Here's how the part is built. I have some questions about the finished solid (model axes, mm). Coordinates: 2 decimals unless noted, no trailing zeros. Write each loop counter-clockwise with the first axis right and the second up, starting at its lowest first coordinate (ties: lowest second). Pieces come first, ordered by that corner, then holes. Notation, with made-up numbers: (2.25, 32.25) - (23.25, 32.25) arc R12 cw to (23.25, 37.25) - close; hole circle Ø10 at (25, 4). An arc over 180 degrees is marked (long way). Answer in a Markdown table with one row per item. Add a question column.
Item 1: If I drill on probe 1 along X at (y, z) = (17.5, -1204); probe 2 along Z at (x, y) = (-498, 19); probe 3 along Z at (x, y) = (-171.5, 14.25), over which ranges is the centre line in solid material (lowest first)? Write a range as from..to.
Item 2: Imagine slicing it at D-D (z = -793.5). Please give me the cut outline in (x, y), plus the area to 3 significant figures.
Item 3: Imagine slicing it at B-B (z = -1252.5). Please give me the cut outline in (x, y), plus the area to 3 significant figures.
Item 4: I'm going to push flat-ended pins straight in: pin 1 (5 mm diameter, centred on x = -369.5, y = 3.5, fed in from +Z); pin 2 (6 mm diameter, centred on y = 17, z = -1120.5, fed in from +X); pin 3 (4 mm diameter, centred on y = 12, z = -1167.5, fed in from +X). Where does each tip first touch, or does it pass through?
Item 5: Imagine slicing it at A-A (y = 9.5). Please give me the cut outline in (x, z), plus the area to 3 significant figures.
Item 6: Imagine slicing it at C-C (x = -313). Please give me the cut outline in (y, z), plus the area to 3 significant figures.
from build123d import *

# Parameters (mm, degrees)
BOSS_EXTRUDE2_DEPTH = 20


with BuildPart() as part:
    # Sketch1 → Boss-Extrude2 (new body)
    with BuildSketch(Plane(origin=(0, 0, 0), x_dir=(1, 0, 0), z_dir=(0, 1, 0))):
        with BuildLine():
            Line((590, 0), (194.448637287, 0))
            ThreePointArc((194.448637287, 0), (189.448637287, -1.339745962), (185.788383249, -5))
            Line((185.788383249, -5), (-144.675037911, -577.379435493))
            ThreePointArc((-144.675037911, -577.379435493), (-150.747101498, -582.038693755), (-158.335291949, -581.03968953))
            Line((-158.335291949, -581.03968953), (-595, -328.931202792))
            ThreePointArc((-595, -328.931202792), (-598.660254038, -325.270948754), (-600, -320.270948754))
            Line((-600, -320.270948754), (-600, 0))
            Line((-600, 0), (-600, 567.320508076))
            ThreePointArc((-600, 567.320508076), (-599.659258263, 569.908698527), (-598.660254038, 572.320508076))
            Line((-598.660254038, 572.320508076), (-123.686027919, 1395))
            ThreePointArc((-123.686027919, 1395), (-120.025773881, 1398.660254038), (-115.025773881, 1400))
            Line((-115.025773881, 1400), (-85, 1400))
            ThreePointArc((-85, 1400), (-77.928932188, 1397.071067812), (-75, 1390))
            Line((-75, 1390), (-75, 1210))
            ThreePointArc((-75, 1210), (-72.071067812, 1202.928932188), (-65, 1200))
            Line((-65, 1200), (65, 1200))
            ThreePointArc((65, 1200), (72.071067812, 1202.928932188), (75, 1210))
            Line((75, 1210), (75, 1390))
            ThreePointArc((75, 1390), (77.928932188, 1397.071067812), (85, 1400))
            Line((85, 1400), (115.025773881, 1400))
            ThreePointArc((115.025773881, 1400), (120.025773881, 1398.660254038), (123.686027919, 1395))
            Line((123.686027919, 1395), (598.660254038, 572.320508076))
            ThreePointArc((598.660254038, 572.320508076), (599.659258263, 569.908698527), (600, 567.320508076))
            Line((600, 567.320508076), (600, 10))
            ThreePointArc((600, 10), (597.071067812, 2.928932188), (590, 0))
        make_face()
    extrude(amount=BOSS_EXTRUDE2_DEPTH)


solid = part.part
Here are the results:
| question | item | result |
|---|---|---|
| 1 | probe 1 | x = -233.96..-73, 73..233.96 |
| 1 | probe 2 | z = -746.67..384.93 |
| 1 | probe 3 | z = -1312.18..573.44 |
| 2 | outline | (-470.96, 0) - (470.96, 0) - (470.96, 20) - (-470.96, 20) - close |
| 2 | area | 18,800 mm2 |
| 3 | outline | (-205.96, 0) - (-75, 0) - (-75, 20) - (-205.96, 20) - close; (75, 0) - (205.96, 0) - (205.96, 20) - (75, 20) - close |
| 3 | area | 5,240 mm2 |
| 4 | pin 1 | stops at z = 460.57 |
| 4 | pin 2 | stops at x = 283.9 |
| 4 | pin 3 | stops at x = 256.19 |
| 5 | outline | (-600, -567.32) arc R10 ccw to (-598.66, -572.32) - (-123.69, -1395) arc R10 ccw to (-115.03, -1400) - (-85, -1400) arc R10 ccw to (-75, -1390) - (-75, -1210) arc R10 cw to (-65, -1200) - (65, -1200) arc R10 cw to (75, -1210) - (75, -1390) arc R10 ccw to (85, -1400) - (115.03, -1400) arc R10 ccw to (123.69, -1395) - (598.66, -572.32) arc R10 ccw to (600, -567.32) - (600, -10) arc R10 ccw to (590, 0) - (194.45, 0) arc R10 cw to (185.79, 5) - (-144.68, 577.38) arc R10 ccw to (-158.34, 581.04) - (-595, 328.93) arc R10 ccw to (-600, 320.27) - close |
| 5 | area | 1,560,000 mm2 |
| 6 | outline | (0, -1067.1) - (20, -1067.1) - (20, 491.74) - (0, 491.74) - close |
| 6 | area | 31,200 mm2 |
